Build history of the part. All positions in model axes, mm. A direction names the side the tool comes from. Give positions to 0.01 mm unless a question says otherwise; leave off trailing zeros. Write each loop counter-clockwise with the first axis right and the second up, starting at its lowest first coordinate (ties: lowest second). Pieces come first, ordered by that corner, then holes. Notation, with made-up numbers: (54, 82.25) -> (85, 82.25) arc R27 cw to (85, 118.25) -> close; hole circle Ø1 at (-10, 4). An arc over 180 degrees is marked (long way). Put each result on its own line as item: value. Start each with the question number.
Item 1: Slice it at B-B, the plane x = 50.5. List the corners of the cut face in (y, z), plus the area to 4 significant figures.
Item 2: Drill centre lines: line 1 along Y through (x, z) = (49.5, -9.5); line 2 along Y through (x, z) = (88, -4.75); line 3 along Y through (x, z) = (66.5, -9.75). Where is each one in solid material? Low to high.
Item 3: Slice it at A-A, the plane x = 65. List the corners of the cut face in (y, z), plus the area to 3 significant figures.
Item 4: Slice it at C-C, the plane y = -39. List the corners of the cut face in (x, z), plus the area to 3 significant figures.
Item 5: Tool access for faces 1 (the flat face through (0.1, 10.2, 0)), 2 (the flat face through (-6.693, 25.796, -8.979)): list every direction of +Z, -Z, +X, -X, +Y, -Y with a clear straight run to the whole face (end or side of a thin tool).
Item 6: Two-plate mould, pull along X, no slides. Class faces 3 (the cylindrical face through (-49.793, 4.544, -6.409)), 4 (the flat face through (65.1, 10.2, 0)), 5 (the flat face through (92.5, -5, -5)): pulls with the +X half, pulls with the -X half, needs draft (parallel to the pull), parting line crosses it, or undercut.
Item 7: Flat gauge pins, fed straight in: pin 1 Ø6 at (x, y) = (30.5, 30) entering from +Z; pin 2 Ø1 at (x, z) = (6, -7.5) entering from -Y; pin 3 Ø17 at (x, y) = (-17, -14) entering from +Z. Where does each tip first touch, or does it go through?
Item 8: Slice it at D-D, the plane y = 35.5. List the corners of the cut face in (x, z).
```python
from build123d import *

# Parameters (mm, degrees)
SKETCH1_R        = 10
SKETCH1_R_2      = 2.5
EXTRUDE1_DEPTH   = 13
SHELL1_START     = -10.5
SHELL1_OUTLINE_R = 12.5
SHELL1_DEPTH     = 10.5
RIB1_REACH       = 109.616
SKETCH2_WALLS_W  = 262.2324325
SKETCH2_WALLS_H  = 4


# Read off the part's stored shape, not the designer's step: Shell1
with BuildPart() as part:
    # Sketch1 → Extrude1 (new body)
    with BuildSketch(Plane.XY):
        with BuildLine():
            Line((43.301270189, 25), (88, 25))
            ThreePointArc((88, 25), (92.949747468, 22.949747468), (95, 18))
            Line((95, 18), (95, -28))
            ThreePointArc((95, -28), (92.949747468, -32.949747468), (88, -35))
            Line((88, -35), (35.707142143, -35))
            ThreePointArc((35.707142143, -35), (-49.604256922, 6.278351312), (43.301270189, 25))
        make_face()
        Circle(SKETCH1_R, mode=Mode.SUBTRACT)
        with Locations((65, 0)):
            Circle(SKETCH1_R, mode=Mode.SUBTRACT)
        with Locations((-8, 44.283179651)):
            Circle(SKETCH1_R_2, mode=Mode.SUBTRACT)
        with Locations((-42.350358538, 15.213386595)):
            Circle(SKETCH1_R_2, mode=Mode.SUBTRACT)
        with Locations((-34.350358538, -29.069793056)):
            Circle(SKETCH1_R_2, mode=Mode.SUBTRACT)
        with Locations((88, 18)):
            Circle(SKETCH1_R_2, mode=Mode.SUBTRACT)
        with Locations((88, -28)):
            Circle(SKETCH1_R_2, mode=Mode.SUBTRACT)
    extrude(amount=-EXTRUDE1_DEPTH)

    # Shell1 outline → Shell1 (cut)
    with BuildSketch(Plane.XY.offset(SHELL1_START)):
        with BuildLine():
            ThreePointArc((-43.004716488, 20.170383234), (-37.644763145, 13.523010307), (-46.009463032, 11.805901554))
            ThreePointArc((-46.009463032, 11.805901554), (-46.743356298, -8.444444445), (-38.970422528, -27.157985344))
            ThreePointArc((-38.970422528, -27.157985344), (-30.533652034, -25.83981605), (-33.228942177, -33.942413023))
            ThreePointArc((-33.228942177, -33.942413023), (1.009270558, -47.489276399), (34.641016151, -32.5))
            Line((34.641016151, -32.5), (85.820550528, -32.5))
            ThreePointArc((85.820550528, -32.5), (84.464466094, -24.464466094), (92.5, -25.820550528))
            Line((92.5, -25.820550528), (92.5, 15.820550528))
            ThreePointArc((92.5, 15.820550528), (84.464466094, 14.464466094), (85.820550528, 22.5))
            Line((85.820550528, 22.5), (41.833001327, 22.5))
            ThreePointArc((41.833001327, 22.5), (22.611889377, 41.772628105), (-4.03429396, 47.328368578))
            ThreePointArc((-4.03429396, 47.328368578), (-7.111111111, 39.362826356), (-12.780520855, 45.748314577))
            ThreePointArc((-12.780520855, 45.748314577), (-30.684781559, 36.25871179), (-43.004716488, 20.170383234))
        make_face()
        Circle(SHELL1_OUTLINE_R, mode=Mode.SUBTRACT)
        with Locations((65, 0)):
            Circle(SHELL1_OUTLINE_R, mode=Mode.SUBTRACT)
    extrude(amount=SHELL1_DEPTH, mode=Mode.SUBTRACT)

    # Sketch2 walls → Rib1 (add, up to next)
    with BuildSketch(Plane.XY.offset(-7.5), mode=Mode.PRIVATE) as rib1_sk1:
        Polygon((-29.277690873, 150.813655589), (15.56363046, -97.40088046), (19.499913096, -96.689769349), (-25.341408238, 151.5247667), align=None)
    rib1_tool1 = extrude(rib1_sk1.sketch, amount=-RIB1_REACH, mode=Mode.PRIVATE) - part.part
    # Sketch2 walls → Rib1 (add, up to next)
    with BuildSketch(Plane.XY.offset(-7.5), mode=Mode.PRIVATE) as rib1_sk2:
        Polygon((93.48575309, -31.457464562), (-143.895001384, 53.816080049), (-145.247302414, 50.051603734), (92.133452059, -35.221940877), align=None)
    rib1_tool2 = extrude(rib1_sk2.sketch, amount=-RIB1_REACH, mode=Mode.PRIVATE) - part.part
    # Sketch2 walls → Rib1 (add, up to next)
    with BuildSketch(Plane.XY.offset(-7.5), mode=Mode.PRIVATE) as rib1_sk3:
        Polygon((-115.969611541, -100.762051855), (76.569821599, 62.178939584), (73.985839994, 65.232304787), (-118.553593146, -97.708686652), align=None)
    rib1_tool3 = extrude(rib1_sk3.sketch, amount=-RIB1_REACH, mode=Mode.PRIVATE) - part.part
    # Sketch2 walls → Rib1 (add, up to next)
    with BuildSketch(Plane.XY.offset(-7.5), mode=Mode.PRIVATE) as rib1_sk4:
        with Locations((32.5, 0)):
            Rectangle(SKETCH2_WALLS_W, SKETCH2_WALLS_H)
    rib1_tool4 = extrude(rib1_sk4.sketch, amount=-RIB1_REACH, mode=Mode.PRIVATE) - part.part
    # Sketch2 walls → Rib1 (add, up to next)
    with BuildSketch(Plane.XY.offset(-7.5), mode=Mode.PRIVATE) as rib1_sk5:
        Polygon((-11.428146954, -62.35299881), (174.768430011, 83.366061423), (172.303196964, 86.516081427), (-13.893380001, -59.202978806), align=None)
    rib1_tool5 = extrude(rib1_sk5.sketch, amount=-RIB1_REACH, mode=Mode.PRIVATE) - part.part
    # Sketch2 walls → Rib1 (add, up to next)
    with BuildSketch(Plane.XY.offset(-7.5), mode=Mode.PRIVATE) as rib1_sk6:
        Polygon((0.858947254, 74.933860572), (155.397541961, -113.20008081), (158.488446979, -110.661123117), (3.949852272, 77.472818265), align=None)
    rib1_tool6 = extrude(rib1_sk6.sketch, amount=-RIB1_REACH, mode=Mode.PRIVATE) - part.part
    add(rib1_tool1.solids().sort_by_distance((-4.888888889, 27.06194312, -7.5))[0])
    add(rib1_tool2.solids().sort_by_distance((-25.880774662, 9.297069586, -7.5))[0])
    add(rib1_tool3.solids().sort_by_distance((-20.991885773, -17.764873534, -7.5))[0])
    add(rib1_tool4.solids().sort_by_distance((32.5, 0, -7.5))[0])
    add(rib1_tool5.solids().sort_by_distance((80.437525005, 12.081541308, -7.5))[0])
    add(rib1_tool6.solids().sort_by_distance((79.673697117, -17.863631273, -7.5))[0])


solid = part.part
```
Values follow:
1. outline: (-35, -13) -> (25, -13) -> (25, 0) -> (22.5, 0) -> (22.5, -10.5) -> (2, -10.5) -> (2, -7.5) -> (-2, -7.5) -> (-2, -10.5) -> (-32.5, -10.5) -> (-32.5, 0) -> (-35, 0) -> close
1. area: 214.5 mm2
2. line 1: -35 to -32.5, -2 to 2, 22.5 to 25
2. line 2: -35 to -30.5, -25.5 to -23, 13 to 15.5, 20.5 to 25
2. line 3: -35 to -32.5, -12.41 to -9.89, 9.89 to 12.41, 22.5 to 25
3. outline: (-35, -13) -> (-10, -13) -> (-10, 0) -> (-12.5, 0) -> (-12.5, -10.5) -> (-32.5, -10.5) -> (-32.5, 0) -> (-35, 0) -> close; (10, -13) -> (25, -13) -> (25, 0) -> (22.5, 0) -> (22.5, -10.5) -> (12.5, -10.5) -> (12.5, 0) -> (10, 0) -> close
3. area: 205 mm2
4. outline: (-31.29, -13) -> (31.29, -13) -> (31.29, 0) -> (27.12, 0) -> (27.12, -10.5) -> (-27.12, -10.5) -> (-27.12, 0) -> (-31.29, 0) -> close
4. area: 244 mm2
5. face 1: +Z, +X, -X, +Y, -Y
5. face 2: +Z
6. face 3: parting line crosses it
6. face 4: needs draft
6. face 5: undercut
7. pin 1: z = -10.5
7. pin 2: y = -49.7
7. pin 3: z = -7.5
8. outline: (-35.21, -13) -> (35.21, -13) -> (35.21, 0) -> (31.56, 0) -> (31.56, -10.5) -> (-4.38, -10.5) -> (-4.38, -7.5) -> (-8.45, -7.5) -> (-8.45, -10.5) -> (-31.56, -10.5) -> (-31.56, 0) -> (-35.21, 0) -> close
